The figure shows three views and two pictorial views of one solid part (mm, origin at its lowest corner). Answer the questions. A direction names the side the tool comes from. Round coordinates to 2 decimals unless told otherwise and drop trailing zeros. Write each loop counter-clockwise with the first axis right and the second up, starting at its lowest first coordinate (ties: lowest second). Pieces come first, ordered by that corner, then holes.
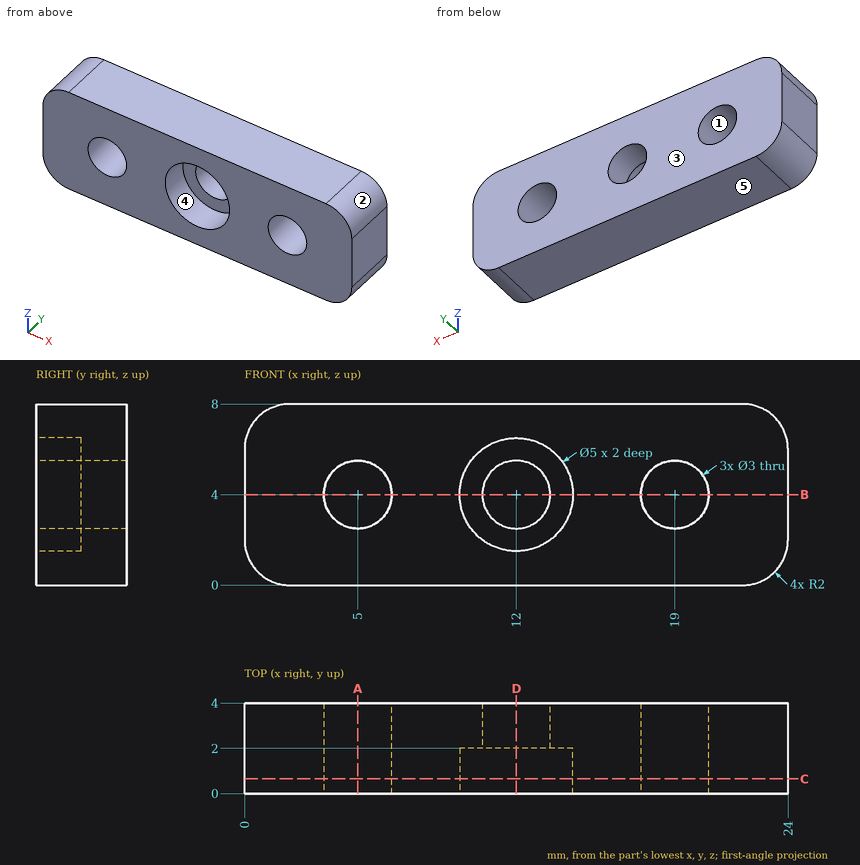
Q1. Section D-D (x = 12) is taken. Determine the outline of the cut face in (y, z), then the cut area to 3 significant figures.
Verdict:
outline: (0, 0) - (4, 0) - (4, 2.5) - (2, 2.5) - (2, 1.5) - (0, 1.5) - close; (0, 6.5) - (2, 6.5) - (2, 5.5) - (4, 5.5) - (4, 8) - (0, 8) - close
area: 16.0 mm2
Q2. Section A-A (x = 5) is taken. Determine the outline of the cut face in (y, z), then the cut area to 3 significant figures.
Verdict:
outline: (0, 0) - (4, 0) - (4, 2.5) - (0, 2.5) - close; (0, 5.5) - (4, 5.5) - (4, 8) - (0, 8) - close
area: 20.0 mm2
Q3. Which of the six approach directions +Z, -Z, +X, -X, +Y, -Y give full straight-line access (tool end or side, diameter ignored) to the marked faces 4 and 5?
Verdict:
face 4: -Y
face 5: -Z, +X, -X, +Y, -Y
Q4. Straight lines are drawn through the part: probe 1 along X at (y, z) = (1.9, 4); probe 2 along X at (y, z) = (1.2, 6); probe 3 along X at (y, z) = (2.85, 5.25). For each, find the intervals that lie inside material, in ascending order.
Verdict:
probe 1: x = 0 to 3.5, 6.5 to 9.5, 14.5 to 17.5, 20.5 to 24
probe 2: x = 0 to 10.5, 13.5 to 24
probe 3: x = 0 to 4.17, 5.83 to 11.17, 12.83 to 18.17, 19.83 to 24
Q5. Flat-ended cylindrical pins translate along their axes: pin 1 Ø1.5 at (x, z) = (11.5, 3.5) entering from -Y; pin 2 Ø4 at (x, z) = (12, 4) entering from -Y; pin 3 Ø3.5 at (x, z) = (5, 4) entering from +Y; pin 4 Ø1 at (y, z) = (3, 1) entering from +X. Find the tip coordinate at first contact, or state that the pin passes through.
Verdict:
pin 1: passes through
pin 2: stops at y = 2
pin 3: stops at y = 4
pin 4: stops at x = 23.94
Q6. Determine the mould class of the marked faces 1, 2 and 3 for opening direction Z: pulls with the +Z half, pulls with the -Z half, needs draft (parallel to the pull), parting line crosses it, or undercut.
Verdict:
face 1: undercut
face 2: pulls with the +Z half
face 3: needs draft
Q7. Section C-C (y = 0.65) is taken. Determine the outline of the cut face in (x, z).
Verdict:
outline: (0, 2) arc R2 ccw to (2, 0) - (22, 0) arc R2 ccw to (24, 2) - (24, 6) arc R2 ccw to (22, 8) - (2, 8) arc R2 ccw to (0, 6) - close; hole circle Ø3 at (5, 4); hole circle Ø5 at (12, 4); hole circle Ø3 at (19, 4)
Q8. Section B-B (z = 4) is taken. Determine the outline of the cut face in (x, y).
Verdict:
outline: (0, 0) - (3.5, 0) - (3.5, 4) - (0, 4) - close; (6.5, 0) - (9.5, 0) - (9.5, 2) - (10.5, 2) - (10.5, 4) - (6.5, 4) - close; (13.5, 2) - (14.5, 2) - (14.5, 0) - (17.5, 0) - (17.5, 4) - (13.5, 4) - close; (20.5, 0) - (24, 0) - (24, 4) - (20.5, 4) - close
